Could you check a few things on this model? Use its own coordinates, in mm. A direction names the side the tool comes from. Round coordinates to 2 decimals unless told otherwise and drop trailing zeros. Loops run counter-clockwise (first coordinate to the right, second up) from the corner with the lowest first, then second, coordinate; pieces in that order, holes last. Notation, with made-up numbers: (-0.5, -23.75) - (50.5, -23.75) arc R23 cw to (50.5, 2.25) - close; hole circle Ø2 at (-36.75, -24.75). An arc over 180 degrees is marked (long way). Use one line per item in the form item = value.
Autodesk Inventor part; units mm, degrees
ref_plane "YZ Plane" through (0, 0, 0) normal (1, 0, 0) x (0, 1, 0)
ref_plane "XZ Plane" through (0, 0, 0) normal (0, 1, 0) x (-1, 0, 0)
ref_plane "XY Plane" through (0, 0, 0) normal (0, 0, 1) x (1, 0, 0)
sketch "Sketch1" plane through (0, 0, 0) normal (0, 1, 0) x (-1, 0, 0)
  circle A0 centre (0, 0) radius 4.125
  dimension "d0" = 8.25
extrude "Extrusion1" add sketch "Sketch1" along normal blind 13
sketch "Sketch2" plane through (0, 0, 0) normal (0, -1, 0) x (1, 0, 0)
  circle A0 centre (0, 0) radius 1
  dimension "d3" = 2
extrude "Extrusion2" cut sketch "Sketch2" against normal blind 8
sketch "Sketch3" plane through (0, 13, 0) normal (0, 1, 0) x (1, 0, 0)
  line L0 (-2.7, -1.2) -> (2.7, -1.2)
  line L1 (2.7, -1.2) -> (2.7, 1.2)
  line L2 (2.7, 1.2) -> (-2.7, 1.2)
  line L3 (-2.7, 1.2) -> (-2.7, -1.2)
  line L4 (-2.7, -1.2) -> (2.7, 1.2) construction
  line L5 (2.7, -1.2) -> (-2.7, 1.2) construction
  point P0 (0, 0)
  dimension "d6" = 2.4
  dimension "d7" = 5.4
extrude "Extrusion3" cut sketch "Sketch3" against normal blind 5
properties part number "encoder_magnet_holder_3DPrint"
1. On a 3-axis mill with a long thin cutter (end or side, diameter ignored), from which of +Z, -Z, +X, -X, +Y, -Y can I reach the whole of each face in a straight line? I mean faces 1 (the face through (0, 4, -1)), 2 (the face through (-2.7, 11, 0)). Say none if no direction works.
Solution:
face_1 = +Y, -Y
face_2 = +Y
2. If we section it at D-D, the plane x = 1.75: Write out the boundary of the cut face in (y, z).
Solution:
outline = (0, -3.74) - (13, -3.74) - (13, -1.2) - (8, -1.2) - (8, 1.2) - (13, 1.2) - (13, 3.74) - (0, 3.74) - close
3. We'd pull the mould along X, two halves only. Please class faces 3 (the face through (-1, 8, -1)), 4 (the face through (-3.8, 6.4, 1.6)), 5 (the face through (0, 13, -2)): +X half, -X half, draft (parallel to the pull), parting line (faces both ways), or undercut.
Solution:
face_3 = undercut
face_4 = parting line
face_5 = draft
4. Please list where these lines run through material, in increasing order: line 1 along Z through (x, y) = (0, 3.5) (3 decimals); line 2 along Z through (x, y) = (2, 12.5); line 3 along Y through (x, z) = (2.25, 0.25).
Solution:
line_1 = -4.125 to -1, 1 to 4.125
line_2 = -3.61 to -1.2, 1.2 to 3.61
line_3 = 0 to 8
5. If we section it at B-B, the plane z = -0.75: Write out the boundary of the cut face in (x, y).
Solution:
outline = (-4.06, 0) - (-0.66, 0) - (-0.66, 8) - (-2.7, 8) - (-2.7, 13) - (-4.06, 13) - close; (0.66, 0) - (4.06, 0) - (4.06, 13) - (2.7, 13) - (2.7, 8) - (0.66, 8) - close
6. If we section it at A-A, the plane x = 0: Write out the boundary of the cut face in (y, z) (3 decimals), plus the area to 4 significant figures.
Solution:
outline = (0, -4.125) - (13, -4.125) - (13, -1.2) - (8, -1.2) - (8, -1) - (0, -1) - close; (0, 1) - (8, 1) - (8, 1.2) - (13, 1.2) - (13, 4.125) - (0, 4.125) - close
area = 79.25 mm^2
7. For P1, Ø1, axis at y = 11, z = 1, coming from the +X side; P2, Ø1, axis at x = -1.5, y = 2, coming from the +Z side, each with a flat end and sliding along its axis, tell me the tip position at first contact or that it passes through.
Solution:
P1 = 4.09
P2 = 4
8. If we section it at C-C, the plane y = 11.75: Write out the boundary of the cut face in (x, z) (3 decimals), plus the area to 3 significant figures.
Solution:
outline = circle Ø8.25 at (0, 0); hole (-2.7, -1.2) - (2.7, -1.2) - (2.7, 1.2) - (-2.7, 1.2) - close
area = 40.5 mm^2
